Source: three-view drawing plus pictorial views. Frame: mm from the lowest corner of the part. A direction names the side the tool comes from. Round coordinates to 2 decimals unless told otherwise and drop trailing zeros. Write each loop counter-clockwise with the first axis right and the second up, starting at its lowest first coordinate (ties: lowest second). Pieces come first, ordered by that corner, then holes. Notation, with made-up numbers: (25.25, 31.25) -> (40.25, 31.25) arc R26 cw to (40.25, 64.25) -> close; hole circle Ø4 at (86.5, 27). An arc over 180 degrees is marked (long way). Put each result on its own line as item: value.
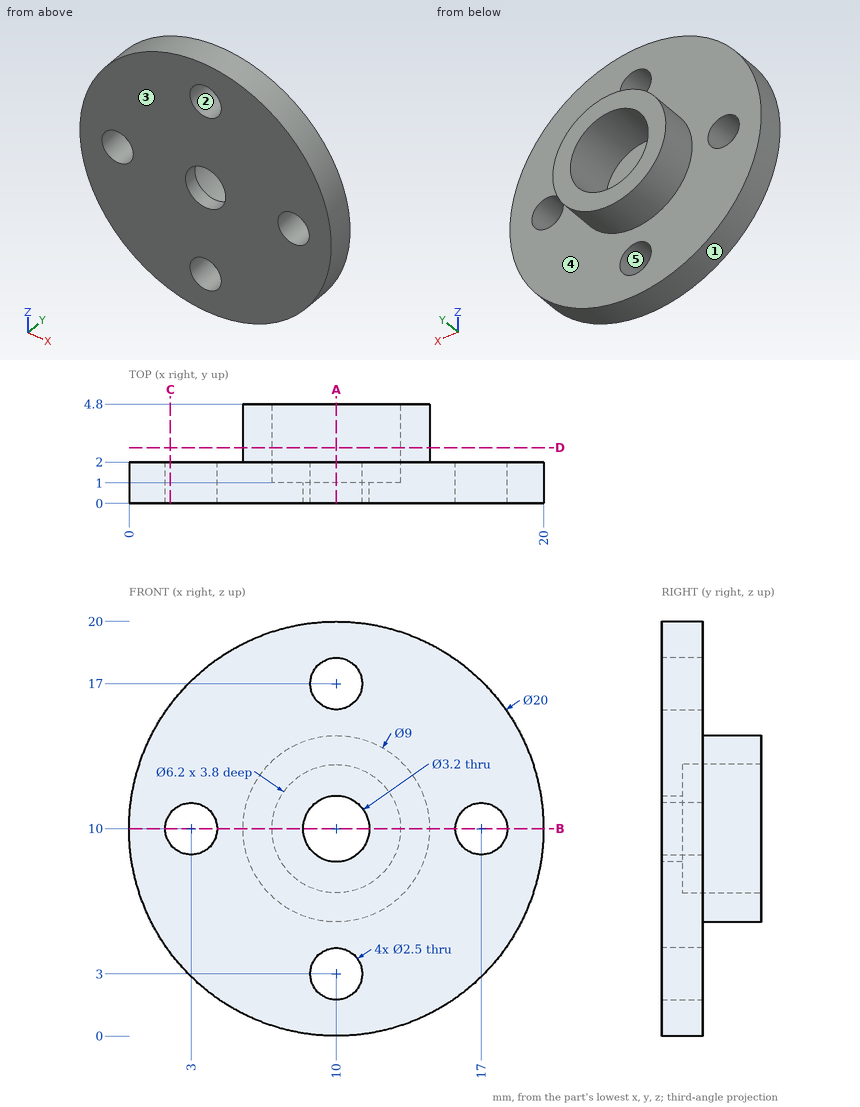
Q1. Pin query (flat end, axial travel): pin 1 (1.5 mm diameter, centred on x = 13.5, y = 3.5, fed in from +Z); pin 2 (4 mm diameter, centred on x = 3, z = 10, fed in from +Y); pin 3 (1.5 mm diameter, centred on x = 17, y = 2.5, fed in from +Z). Return the tip coordinate at first contact, or that it passes through.
Ans:
pin 1: stops at z = 13.56
pin 2: stops at y = 2
pin 3: stops at z = 17.65
Q2. Material intervals for line 1 (X direction, y = 0.7, z = 10); line 2 (X direction, y = 3.6, z = 10); line 3 (Y direction, x = 16, z = 4), sorted ascending. Write a range as [from, to].
Ans:
line 1: x = [0, 1.75], [4.25, 8.4], [11.6, 15.75], [18.25, 20]
line 2: x = [5.5, 6.9], [13.1, 14.5]
line 3: y = [0, 2]
Q3. Draft query along X for the marked faces 1, 2 and 3. Return one class per face: +X half, -X half, draft (parallel to the pull), parting line (faces both ways), or undercut.
Ans:
face 1: parting line
face 2: undercut
face 3: draft
Q4. Reachability of the marked faces 4 and 5 from +Z, -Z, +X, -X, +Y, -Y: full face, straight path, thin tool, end or side. Return the list, or none.
Ans:
face 4: +Y
face 5: +Y, -Y
Q5. Cut plane C-C on x = 2. Output: boundary loops of the cut face in (y, z), and give its area (3 significant figures).
Ans:
outline: (0, 4) -> (2, 4) -> (2, 9.25) -> (0, 9.25) -> close; (0, 10.75) -> (2, 10.75) -> (2, 16) -> (0, 16) -> close
area: 21.0 mm^2
Q6. Cut plane A-A on x = 10. Output: boundary loops of the cut face in (y, z).
Ans:
outline: (0, 0) -> (2, 0) -> (2, 1.75) -> (0, 1.75) -> close; (0, 4.25) -> (2, 4.25) -> (2, 5.5) -> (4.8, 5.5) -> (4.8, 6.9) -> (1, 6.9) -> (1, 8.4) -> (0, 8.4) -> close; (0, 11.6) -> (1, 11.6) -> (1, 13.1) -> (4.8, 13.1) -> (4.8, 14.5) -> (2, 14.5) -> (2, 15.75) -> (0, 15.75) -> close; (0, 18.25) -> (2, 18.25) -> (2, 20) -> (0, 20) -> close
Q7. Cut plane B-B on z = 10. Output: boundary loops of the cut face in (x, y), and give its area (3 significant figures).
Ans:
outline: (0, 0) -> (1.75, 0) -> (1.75, 2) -> (0, 2) -> close; (4.25, 0) -> (8.4, 0) -> (8.4, 1) -> (6.9, 1) -> (6.9, 4.8) -> (5.5, 4.8) -> (5.5, 2) -> (4.25, 2) -> close; (11.6, 0) -> (15.75, 0) -> (15.75, 2) -> (14.5, 2) -> (14.5, 4.8) -> (13.1, 4.8) -> (13.1, 1) -> (11.6, 1) -> close; (18.25, 0) -> (20, 0) -> (20, 2) -> (18.25, 2) -> close
area: 28.4 mm^2
Q8. Cut plane D-D on y = 2.7. Output: boundary loops of the cut face in (x, z), and give its area (3 significant figures).
Ans:
outline: circle Ø9 at (10, 10); hole circle Ø6.2 at (10, 10)
area: 33.4 mm^2
